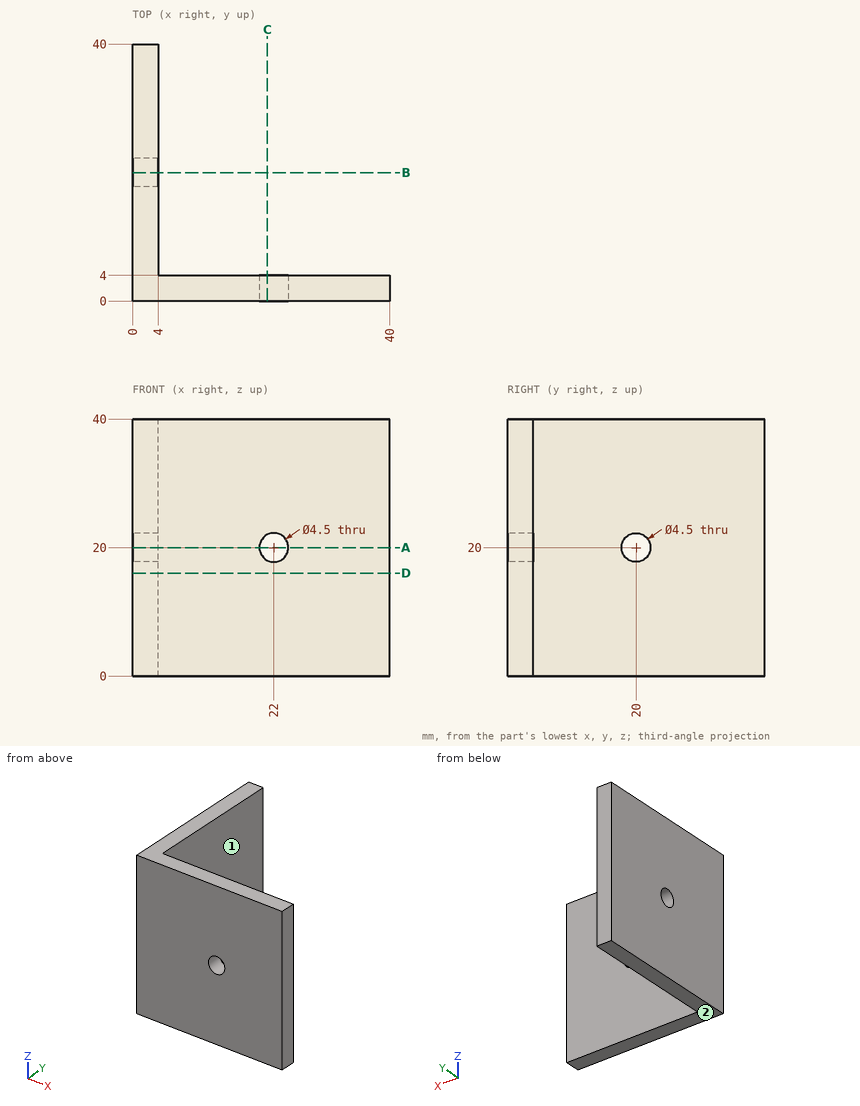
Source: three-view drawing plus pictorial views. Frame: mm from the lowest corner of the part. A direction names the side the tool comes from. Give positions to 0.01 mm unless a question says otherwise; leave off trailing zeros. Order: outer loops, then holes, each group sorted by start corner. A loop starts at its lowest first (then second) coordinate and runs counter-clockwise, first axis right, second up. Notation, with made-up numbers: M 23,5 L 57,5 A25 ccw 57,38 Z; hole C 2.5,-27 d1. An arc over 180 degrees is marked long. Return JSON: item names as keys, results as strings.
1) Line query: L1, parallel to X at y = 2, z = 20; L2, parallel to Y at x = 1.3, z = 20; L3, parallel to X at y = 22, z = 7. Output: solid intervals per line, ascending. Write a range as [from, to].
Taken from the geometry:
{"L1": "x = [0, 19.75], [24.25, 40]", "L2": "y = [0, 17.75], [22.25, 40]", "L3": "x = [0, 4]"}
2) Contact query for flat-ended pins moving along their axis: pin 1 (6 mm diameter, centred on x = 22, z = 20, fed in from +Y); pin 2 (5 mm diameter, centred on y = 20, z = 20, fed in from +X). Output: stop coordinate, or through.
Taken from the geometry:
{"pin 1": "stops at y = 4", "pin 2": "stops at x = 4"}
3) Section query A-A on z = 20. Output: boundary loops of the cut face in (x, y).
Taken from the geometry:
{"outline": "M 0,0 L 19.75,0 L 19.75,4 L 4,4 L 4,17.75 L 0,17.75 Z; M 0,22.25 L 4,22.25 L 4,40 L 0,40 Z; M 24.25,0 L 40,0 L 40,4 L 24.25,4 Z"}
4) Section query B-B on y = 20. Output: boundary loops of the cut face in (x, z).
Taken from the geometry:
{"outline": "M 0,0 L 4,0 L 4,17.75 L 0,17.75 Z; M 0,22.25 L 4,22.25 L 4,40 L 0,40 Z"}
5) Access query for the marked faces 1 and 2. Directions: +Z, -Z, +X, -X, +Y, -Y. A direction counts if a zero-diameter tool reaches every point of the face in a straight line with its end or side. Return the directions, or none.
Taken from the geometry:
{"face 1": "+Z, -Z, +X, +Y", "face 2": "-Z, +X, -X, +Y, -Y"}
6) Section query C-C on x = 21. Output: boundary loops of the cut face in (y, z), and give its area (3 significant figures).
Taken from the geometry:
{"outline": "M 0,0 L 4,0 L 4,17.98 L 0,17.98 Z; M 0,22.02 L 4,22.02 L 4,40 L 0,40 Z", "area": "144 mm2"}
7) Section query D-D on z = 16. Output: boundary loops of the cut face in (x, y), and give its area (3 significant figures).
Taken from the geometry:
{"outline": "M 0,0 L 40,0 L 40,4 L 4,4 L 4,40 L 0,40 Z", "area": "304 mm2"}
